Study the drawing (mm; zero at the part's minimum x, y, z) and answer. Give positions to 0.01 mm unless a question says otherwise; leave off trailing zeros. Order: outer loops, then holes, each group sorted by start corner. A loop starts at its lowest first (then second) coordinate and runs counter-clockwise, first axis right, second up. Notation, with made-up numbers: (69, 88) - (123, 88) arc R21 ccw to (123, 124) - close; hole circle Ø4 at (12, 54.25). An arc over 180 degrees is marked (long way). Put each result on its own line as item: value.
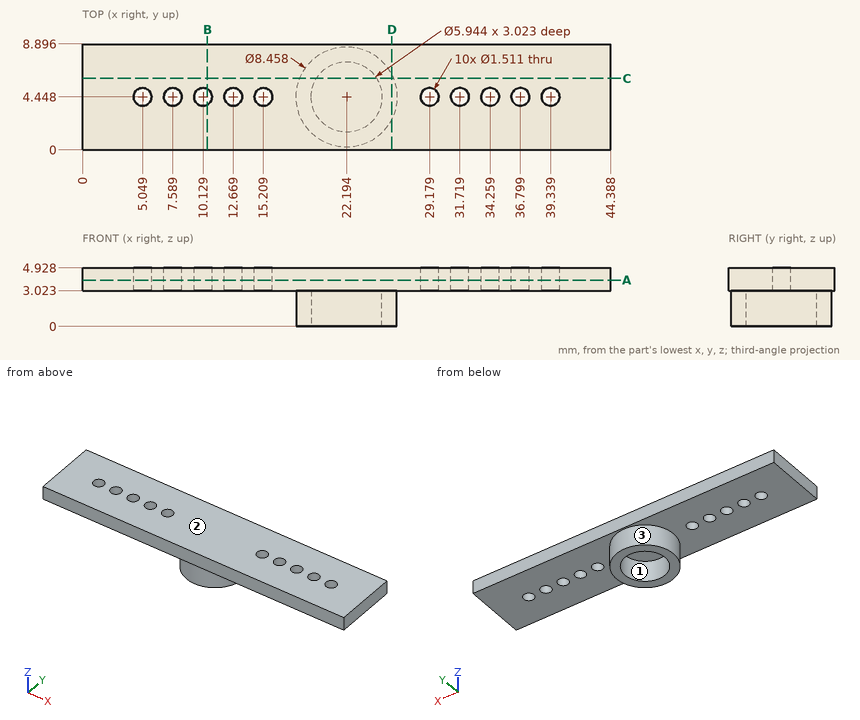
(1) Section D-D, the plane x = 26 is taken. Write down the section's boundary in (y, z) (1 decimal), then the cut area to 3 significant figures.
Geometry check:
outline: (0, 3) - (2.6, 3) - (2.6, 0) - (6.3, 0) - (6.3, 3) - (8.9, 3) - (8.9, 4.9) - (0, 4.9) - close
area: 28.1 mm²
(2) Section B-B, the plane x = 10.5 is taken. Write down the section's boundary in (y, z) (1 decimal).
Geometry check:
outline: (0, 3) - (3.8, 3) - (3.8, 4.9) - (0, 4.9) - close; (5.1, 3) - (8.9, 3) - (8.9, 4.9) - (5.1, 4.9) - close
(3) Straight lines are drawn through the part: line 1 (Y direction, x = 22, z = 1.45); line 2 (Z direction, x = 6.5, y = 1); line 3 (X direction, y = 5.75, z = 1.55) (1 decimal). For each, find the intervals that lie inside material, in ascending order.
Geometry check:
line 1: y = 0.22 to 1.48, 7.41 to 8.67
line 2: z = 3.02 to 4.93
line 3: x = 18.2 to 19.5, 24.9 to 26.2
(4) Determine the mould class of the marked faces 1, 2 and 3 for opening direction X: pulls with the +X half, pulls with the -X half, needs draft (parallel to the pull), parting line crosses it, or undercut.
Geometry check:
face 1: undercut
face 2: needs draft
face 3: parting line crosses it
(5) Section A-A, the plane z = 3.9 is taken. Count the separate pieces of the cut face and the enclosed holes in it, then the cut area to 3 significant figures.
Geometry check:
separate pieces: 1
enclosed holes: 10
area: 377 mm²
(6) Given pin 1 (2 mm diameter, centred on x = 10.13, y = 4.45, fed in from -Z); pin 2 (2 mm diameter, centred on y = 7.5, z = 1, fed in from -X) (1 decimal), each flat-ended and moving along its own axis, determine where each tip first touches the part or whether it passes through.
Geometry check:
pin 1: stops at z = 3.02
pin 2: stops at x = 18.5
(7) Section C-C, the plane y = 6 is taken. Write down the section's boundary in (x, z).
Geometry check:
outline: (0, 3.02) - (18.26, 3.02) - (18.26, 0) - (19.66, 0) - (19.66, 3.02) - (24.73, 3.02) - (24.73, 0) - (26.13, 0) - (26.13, 3.02) - (44.39, 3.02) - (44.39, 4.93) - (0, 4.93) - close
